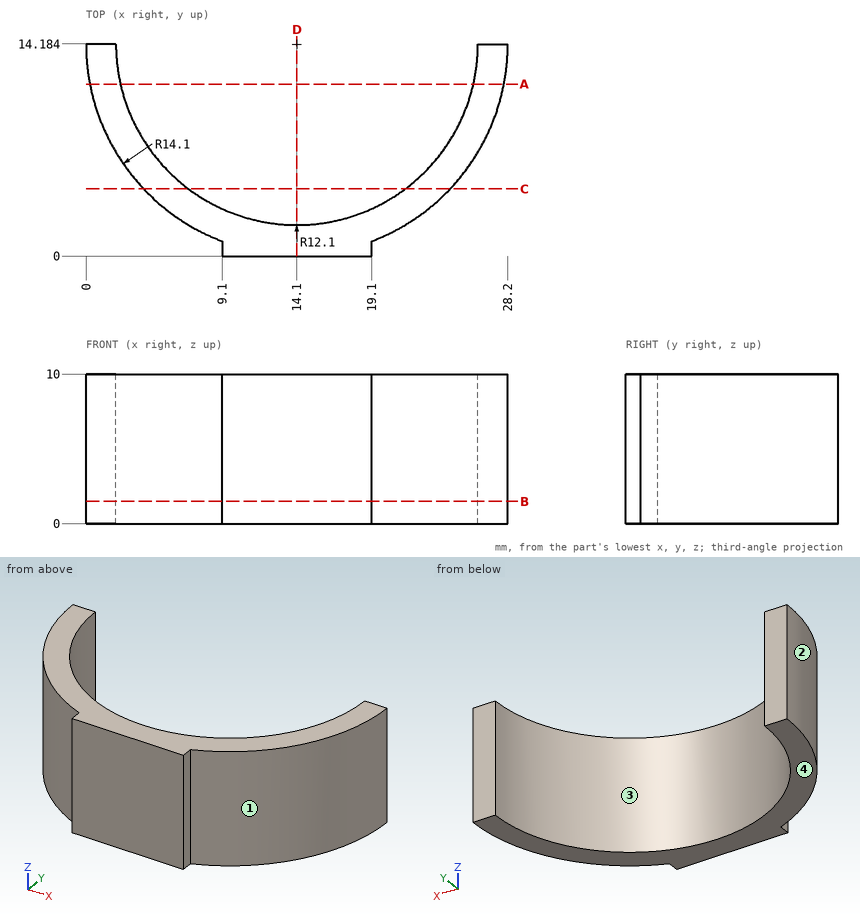
The drawing under review shows one solid part. Ordinate dimensions are in mm from its lowest x, y, z. Coordinates: 2 decimals unless noted, no trailing zeros. Write each loop counter-clockwise with the first axis right and the second up, starting at its lowest first coordinate (ties: lowest second). Pieces come first, ordered by that corner, then holes. Notation, with made-up numbers: (41.25, 72.5) - (67.25, 72.5) arc R9 ccw to (67.25, 85.5) - close; hole circle Ø1 at (30.25, -16.5). An arc over 180 degrees is marked (long way). Use one line per item in the form item = value.
Q1. Consider section C-C (y = 4.5). Write out the cut boundary in (x, z) (1 decimal).
Taken from the geometry:
outline = (3.9, 0) - (6.8, 0) - (6.8, 10) - (3.9, 10) - close; (21.4, 0) - (24.3, 0) - (24.3, 10) - (21.4, 10) - close
Q2. The part is to be moulded in two halves that separate along X. For the marked faces 1, 2, 3 and 4, say which applies: +X half, -X half, draft (parallel to the pull), parting line (faces both ways), or undercut.
Taken from the geometry:
face_1 = +X half
face_2 = -X half
face_3 = undercut
face_4 = draft
Q3. For probe 1 along X at (y, z) = (11.25, 2.25); probe 2 along X at (y, z) = (6.5, 1.25); probe 3 along X at (y, z) = (2, 5.75) (1 decimal), list the stretches that pass through material, from the lowest coordinate up.
Taken from the geometry:
probe_1 = 0.31 to 2.36, 25.84 to 27.89
probe_2 = 2.28 to 4.75, 23.45 to 25.92
probe_3 = 7 to 21.2
Q4. Consider section A-A (y = 11.5). Write out the cut boundary in (x, z).
Taken from the geometry:
outline = (0.26, 0) - (2.3, 0) - (2.3, 10) - (0.26, 10) - close; (25.9, 0) - (27.94, 0) - (27.94, 10) - (25.9, 10) - close
Q5. Insertion check: pin 1 Ø2 at (x, z) = (9.5, 5.5) entering from +Y; pin 2 Ø0.8 at (y, z) = (0.5, 7) entering from -X; pin 3 Ø0.5 at (y, z) = (0.5, 5.5) entering from +X. Each pin has a flat end and moves straight along its axis. Give the tip position at first contact, or say it passes through.
Taken from the geometry:
pin_1 = 3.46
pin_2 = 9.1
pin_3 = 19.1
Q6. Consider section D-D (x = 14.1). Write out the cut boundary in (y, z).
Taken from the geometry:
outline = (0, 0) - (2.08, 0) - (2.08, 10) - (0, 10) - close
Q7. Consider section B-B (z = 1.5). Write out the cut boundary in (x, y).
Taken from the geometry:
outline = (0, 14.18) arc R14.1 ccw to (9.1, 1) - (9.1, 0) - (19.1, 0) - (19.1, 1) arc R14.1 ccw to (28.2, 14.18) - (26.2, 14.18) arc R12.1 cw to (2, 14.18) - close
